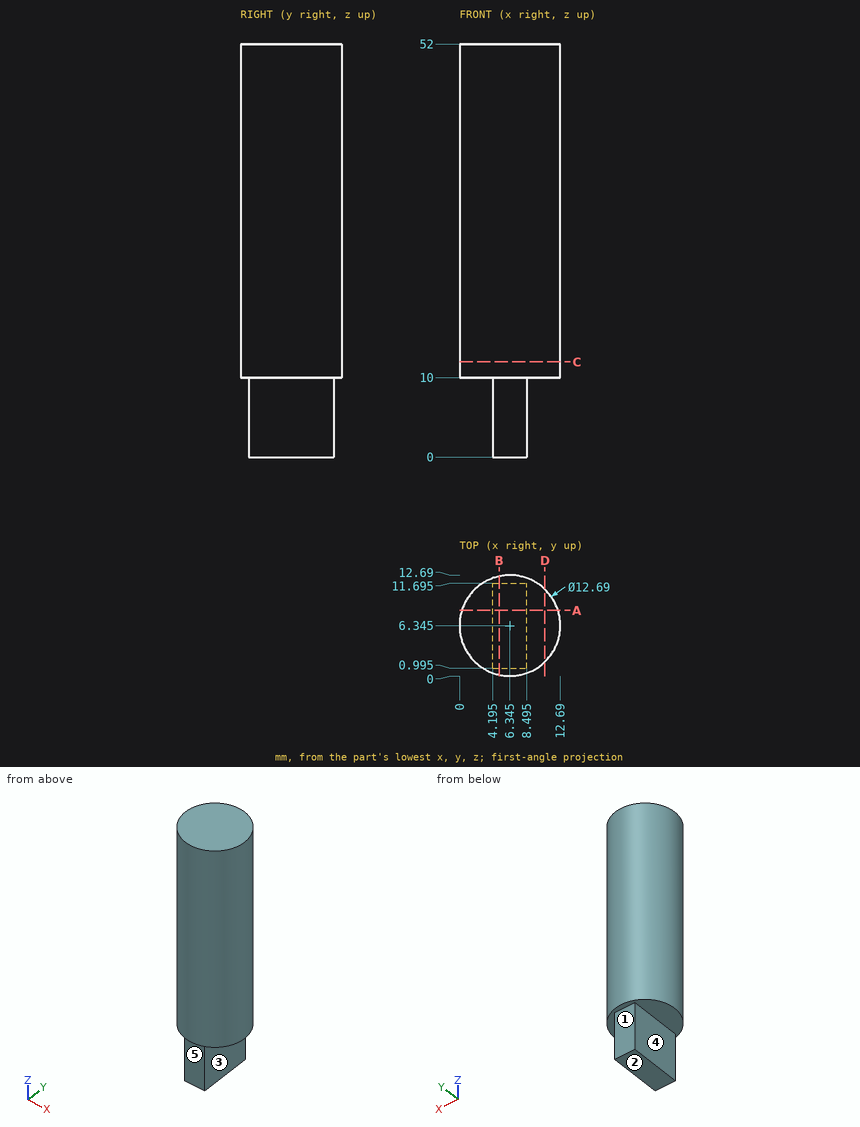
Study the drawing (mm; zero at the part's minimum x, y, z) and answer. A direction names the side the tool comes from. Coordinates: 2 decimals unless noted, no trailing zeros. Write each loop counter-clockwise with the first axis right and the second up, starting at its lowest first coordinate (ties: lowest second). Pieces come first, ordered by that corner, then holes.
Q1. Section D-D, the plane x = 10.75 is taken. Write down the section's boundary in (y, z), then the cut area to 3 significant figures.
Returned:
outline: (1.78, 10) - (10.91, 10) - (10.91, 52) - (1.78, 52) - close
area: 384 mm2
Q2. Section C-C, the plane z = 12 is taken. Write down the section's boundary in (x, y) (3 decimals), then the cut area to 3 significant figures.
Returned:
outline: circle Ø12.69 at (6.345, 6.345)
area: 126 mm2
Q3. Given P1, Ø3, axis at y = 6.5, z = 6.5, coming from the -X side (3 decimals); P2, Ø1.5, axis at y = 10, z = 31, coming from the +X side; P3, Ø5, axis at y = 6, z = 4, coming from the +X side (3 decimals), each flat-ended and moving along its own axis, determine where each tip first touches the part or whether it passes through.
Returned:
P1: stops at x = 4.195
P2: stops at x = 11.99
P3: stops at x = 8.495
Q4. Section B-B, the plane x = 5 is taken. Write down the section's boundary in (y, z) (3 decimals), then the cut area to 3 significant figures.
Returned:
outline: (0.144, 10) - (0.995, 10) - (0.995, 0) - (11.695, 0) - (11.695, 10) - (12.546, 10) - (12.546, 52) - (0.144, 52) - close
area: 628 mm2
Q5. Section A-A, the plane y = 8.25 is taken. Write down the section's boundary in (x, z) (3 decimals), then the cut area to 3 significant figures.
Returned:
outline: (0.293, 10) - (4.195, 10) - (4.195, 0) - (8.495, 0) - (8.495, 10) - (12.397, 10) - (12.397, 52) - (0.293, 52) - close
area: 551 mm2
Q6. Find the intervals of material crossed by line 1 along Z through (x, y) = (9.5, 1); line 2 along X through (y, z) = (3.25, 7.5) (3 decimals); line 3 along X through (y, z) = (6.5, 30.5), in increasing order.
Returned:
line 1: z = 10 to 52
line 2: x = 4.195 to 8.495
line 3: x = 0 to 12.69
Q7. Which of the six approach directions +Z, -Z, +X, -X, +Y, -Y give full straight-line access (tool end or side, diameter ignored) to the marked faces 1, 2, 3, 4 and 5?
Returned:
face 1: -Z, +X, -X, +Y
face 2: -Z, +X, -X, +Y, -Y
face 3: -Z, +X, +Y, -Y
face 4: -Z, -X, +Y, -Y
face 5: -Z, +X, -X, -Y
